from build123d import *

# Parameters (mm, degrees)
SKETCH_1_R          = 1.9
EXTRUDE_1_DEPTH     = 18
CHAMFER_1_SIZE      = 1.5
CHAMFER_1_SIZE2     = 0.3
SKETCH_2_W          = 0.7
SKETCH_2_H          = 3.336204296
CUT_EXTRUDE_1_DEPTH = 18


with BuildPart() as part:
    # 草图1 → 凸台-拉伸1 (new body)
    with BuildSketch(Plane.XY):
        Circle(SKETCH_1_R)
    extrude(amount=EXTRUDE_1_DEPTH)

    # 倒角1
    chamfer_1_edges = [part.edges().sort_by_distance(p)[0] for p in [
        (-1.9, 0, 18),
    ]]
    chamfer_1_side = [part.faces().sort_by_distance(p)[0] for p in [
        (-1.9, 0, 9),
    ]]
    chamfer(chamfer_1_edges, length=CHAMFER_1_SIZE, length2=CHAMFER_1_SIZE2, reference=chamfer_1_side[0])

    # 草图2 → 切除-拉伸1 (cut)
    with BuildSketch(Plane(origin=(0, 0, 0), x_dir=(-1, 0, 0), z_dir=(0, 0, -1))):
        with Locations((-1.9, 0)):
            Rectangle(SKETCH_2_W, SKETCH_2_H)
    extrude(amount=-CUT_EXTRUDE_1_DEPTH, mode=Mode.SUBTRACT)


solid = part.part
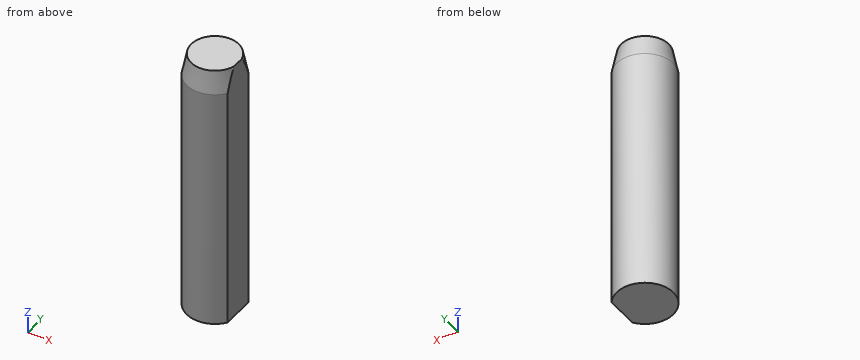
Can you work these out from the model? Positions are in its coordinate system, mm. Coordinates: 2 decimals unless noted, no trailing zeros. Write each loop counter-clockwise with the first axis right and the second up, starting at its lowest first coordinate (ties: lowest second). Pieces come first, ordered by that corner, then holes. Notation, with made-up numbers: (-29.75, 77.5) -> (-6.75, 77.5) arc R33 cw to (-6.75, 108.5) -> close; hole circle Ø7 at (46, -13). An arc over 180 degrees is marked (long way). Write item = value, one per line.
(1) Imagine slicing it at A-A (z = 12.25). Please give me the cut outline in (x, y), and give its area (3 significant figures).
Verdict:
outline = (1.55, -1.1) -> (1.55, 1.1) arc R1.9 ccw (long way) to start
area = 10.8 mm^2
(2) If I drill on probe 1 along X at (y, z) = (1.55, 2.25); probe 2 along X at (y, z) = (1.5, 4.25); probe 3 along Y at (x, z) = (-1.3, 13.5), over which ranges is the centre line in solid material (lowest first)?
Verdict:
probe_1 = -1.1 to 1.1
probe_2 = -1.17 to 1.17
probe_3 = -1.39 to 1.39
(3) For pin 1 (1 mm diameter, centred on x = -1, z = 13, fed in from +Y), with a flat end and sliding along its axis, tell me the tip position at first contact or that it passes through.
Verdict:
pin_1 = 1.83
